from build123d import *

# Parameters (mm, degrees)
F0_R      = 37.5
F0_R_2    = 30
F1_DEPTH  = 4
F2_R      = 1
F3_DEPTH  = 25
F4_R      = 30
F4_R_2    = 27.5
F5_DEPTH  = 4
F6_R      = 30
F8_R      = 23
F11_R     = 27.5
F10_R     = 20.5
F13_R     = 23
F13_R_2   = 15
F14_DEPTH = 2


with BuildPart() as f1:
    # F0 (on Front) → F1 (new body)
    with BuildSketch(Plane.XZ):
        Circle(F0_R)
        Circle(F0_R_2, mode=Mode.SUBTRACT)
    extrude(amount=F1_DEPTH)

    # F2 (on face) → F3 (cut)
    with BuildSketch(Plane.XZ.offset(4)):
        with Locations((0, 33.75)):
            Circle(F2_R)
        with Locations((-33.75, 0)):
            Circle(F2_R)
        with Locations((33.75, 0)):
            Circle(F2_R)
        with Locations((0, -33.75)):
            Circle(F2_R)
    extrude(amount=-F3_DEPTH, mode=Mode.SUBTRACT)

    # F4 (on face) → F5 (join)
    with BuildSketch(Plane(origin=(0, 0, 0), x_dir=(-1, 0, 0), z_dir=(0, 1, 0))):
        Circle(F4_R)
        Circle(F4_R_2, mode=Mode.SUBTRACT)
    extrude(amount=-F5_DEPTH)

    # F6 (on face) → F9 section 0
    with BuildSketch(Plane.XZ.offset(4)):
        Circle(F6_R)
    # F8 (on offset) → F9 section 1
    with BuildSketch(Plane.XZ.offset(42)):
        Circle(F8_R)
    loft()

    # F11 (on face) → F12 section 0
    with BuildSketch(Plane(origin=(0, -4, 0), x_dir=(-1, 0, 0), z_dir=(0, 1, 0))):
        Circle(F11_R)
    # F10 (on face) → F12 section 1
    with BuildSketch(Plane.XZ.offset(42)):
        Circle(F10_R)
    loft(mode=Mode.SUBTRACT)

    # F13 (on face) → F14 (join)
    with BuildSketch(Plane.XZ.offset(42)):
        Circle(F13_R)
        Circle(F13_R_2, mode=Mode.SUBTRACT)
    extrude(amount=F14_DEPTH)


solid = f1.part
Can you work these out from the model? Positions are in its coordinate system, mm. A direction names the side the tool comes from. Coordinates: 2 decimals unless noted, no trailing zeros. Write each loop counter-clockwise with the first axis right and the second up, starting at its lowest first coordinate (ties: lowest second). Pieces come first, ordered by that corner, then holes. Notation, with made-up numbers: (28.25, 21) -> (34.25, 21) arc R22 cw to (34.25, 49) -> close; hole circle Ø5 at (32.5, 72.25). An arc over 180 degrees is marked (long way). Write each question's results on one line, items separated by ' | '. Start each with the question number.
Q1. Imagine slicing it at A-A (x = 0). Write out the boundary of the cut face in (y, z).
Q2. Imagine slicing it at D-D (z = 0). State how many separate pieces and enclosed holes the cut face has, then the cut area to 3 significant figures.
Q3. Imagine slicing it at B-B (z = 33.75). Write out the boundary of the cut face in (x, y), then the cut area to 3 significant figures.
Q4. Imagine slicing it at C-C (x = 33.75). Write out the boundary of the cut face in (y, z).
Q5. I'm going to push flat-ended pins straight in: pin 1 (3 mm diameter, centred on y = -17, z = -21.5, fed in from +X); pin 2 (1.6 mm diameter, centred on x = 0, z = -33.75, fed in from -Y); pin 3 (6 mm diameter, centred on y = -13.5, z = -4.5, fed in from +X); pin 4 (6 mm diameter, centred on x = 20.5, y = -25.5, fed in from -Z). Where does each tip first touch, or does it pass through?
Q6. If I drill on probe 1 along Z at (x, y) = (0, -2.7); probe 2 along Z at (x, y) = (0, -43); probe 3 along Z at (x, y) = (10, -36), over which ranges is the centre line in solid material (lowest first)?
Q7. We'd pull the mould along X, two halves only. Please class faces 4 (the face through (-0.13, -2.03, 34.74)), 5 (the face through (-4.88, -1.97, 37.18)), 6 (the face through (-3, 0, 28)): +X half, -X half, draft (parallel to the pull), parting line (faces both ways), or undercut.
Q8. On a 3-axis mill with a long thin cutter (end or side, diameter ignored), from which of +Z, -Z, +X, -X, +Y, -Y can I reach the whole of each face in a straight line? I mean faces 1 (the face through (5.961, -1.972, -26.846)), 2 (the face through (-14.985, -42.986, 0.66)), 3 (the face through (11.3, -4, 28)). Say none if no direction works.
Taken from the geometry:
1) outline: (-44, -23) -> (-42, -23) -> (-4, -30) -> (-4, -32.75) -> (0, -32.75) -> (0, -27.5) -> (-4, -27.5) -> (-42, -20.5) -> (-42, -15) -> (-44, -15) -> close; (-44, 15) -> (-42, 15) -> (-42, 20.5) -> (-4, 27.5) -> (0, 27.5) -> (0, 32.75) -> (-4, 32.75) -> (-4, 30) -> (-42, 23) -> (-44, 23) -> close; (-4, -37.5) -> (0, -37.5) -> (0, -34.75) -> (-4, -34.75) -> close; (-4, 34.75) -> (0, 34.75) -> (0, 37.5) -> (-4, 37.5) -> close
2) separate pieces: 4 | enclosed holes: 0 | area: 286 mm^2
3) outline: (-16.35, -4) -> (-1, -4) -> (-1, 0) -> (-16.35, 0) -> close; (1, -4) -> (16.35, -4) -> (16.35, 0) -> (1, 0) -> close | area: 123 mm^2
4) outline: (-4, -16.35) -> (0, -16.35) -> (0, -1) -> (-4, -1) -> close; (-4, 1) -> (0, 1) -> (0, 16.35) -> (-4, 16.35) -> close
5) pin 1: stops at x = 19.08 | pin 2: passes through | pin 3: stops at x = 28.57 | pin 4: stops at z = -19.38
6) probe 1: z = -37.5 to -34.75, -32.75 to -27.5, 27.5 to 32.75, 34.75 to 37.5 | probe 2: z = -23 to -15, 15 to 23 | probe 3: z = -21.93 to -19.15, 19.15 to 21.93
7) face 4: undercut | face 5: parting line | face 6: draft
8) face 1: +Y | face 2: +Y, -Y | face 3: -Y
